Could you check a few things on this model? Use its own coordinates, in mm. A direction names the side the tool comes from. Round coordinates to 2 decimals unless told otherwise and drop trailing zeros. Loops run counter-clockwise (first coordinate to the right, second up) from the corner with the lowest first, then second, coordinate; pieces in that order, holes last. Notation, with made-up numbers: (74.5, -3.75) -> (82.5, -3.75) arc R22 ccw to (82.5, 31.25) -> close; hole circle Ø7 at (-22, 61.25). An arc over 180 degrees is marked (long way). Write each question's results on one line, items separated by ' | '.
from build123d import *

# Parameters (mm, degrees)
F1_DEPTH = 10
F2_W     = 8
F2_H     = 1.25
F3_DEPTH = 25
F4_W     = 0.5
F4_H     = 0.5
F5_DEPTH = 25
F6_W     = 6
F6_H     = 1
F7_DEPTH = 1


with BuildPart() as f1:
    # F0 (on Top) → F1 (new body)
    with BuildSketch(Plane.XY):
        Polygon((0, 3.5), (0, 0), (6, 0), (6, 11.5), (5, 11.5), (5, 3.5), align=None)
    extrude(amount=F1_DEPTH)

    # F2 (on face) → F3 (cut)
    with BuildSketch(Plane(origin=(5, 0, 0), x_dir=(0, -1, 0), z_dir=(-1, 0, 0))):
        with Locations((-7.5, 0.625)):
            Rectangle(F2_W, F2_H)
        with Locations((-7.5, 9.375)):
            Rectangle(F2_W, F2_H)
    extrude(amount=-F3_DEPTH, mode=Mode.SUBTRACT)

    # F4 (on face) → F5 (cut)
    with BuildSketch(Plane.XZ):
        with Locations((3.75, 8.5)):
            Rectangle(F4_W, F4_H)
        with Locations((3.75, 1.5)):
            Rectangle(F4_W, F4_H)
        with Locations((3.75, 6.166667)):
            Rectangle(F4_W, F4_H)
        with Locations((3.75, 3.833333)):
            Rectangle(F4_W, F4_H)
    extrude(amount=-F5_DEPTH, mode=Mode.SUBTRACT)

    # F6 (on face) → F7 (cut)
    with BuildSketch(Plane.XZ):
        with Locations((3, 8.5)):
            Rectangle(F6_W, F6_H)
        with Locations((3, 6.166667)):
            Rectangle(F6_W, F6_H)
        with Locations((3, 3.833333)):
            Rectangle(F6_W, F6_H)
        with Locations((3, 1.5)):
            Rectangle(F6_W, F6_H)
    extrude(amount=-F7_DEPTH, mode=Mode.SUBTRACT)


solid = f1.part
1) I want a section at D-D, the plane y = 3.75. Write out the boundary of the cut face in (x, z).
Model answer:
outline: (5, 1.25) -> (6, 1.25) -> (6, 8.75) -> (5, 8.75) -> close
2) I want a section at B-B, the plane z = 7. Write out the boundary of the cut face in (x, y).
Model answer:
outline: (0, 0) -> (6, 0) -> (6, 11.5) -> (5, 11.5) -> (5, 3.5) -> (0, 3.5) -> close
3) I'm going to push flat-ended pins straight in: pin 1 (0.8 mm diameter, centred on x = 5.5, y = 9, fed in from -Z); pin 2 (3 mm diameter, centred on y = 6.5, z = 9, fed in from -X); pin 3 (0.8 mm diameter, centred on x = 4.5, z = 1.5, fed in from -Y). Where does each tip first touch, or does it pass through?
Model answer:
pin 1: stops at z = 1.25 | pin 2: stops at x = 5 | pin 3: stops at y = 1
4) For faces 4 (the flat face through (3, 0.5, 5.667)), 5 (the flat face through (3, 0, 3)), 6 (the flat face through (5.5, 7.6, 8.75)), which set-ups out of +Z, -Z, +X, -X, +Y, -Y let a thin tool reach every point of the face, with its end or its side?
Model answer:
face 4: +X, -X, -Y | face 5: +Z, -Z, +X, -X, -Y | face 6: +Z, +X, -X, +Y
5) If we mould it in two halves opening along Z, with no side actions, what happens to faces 1 (the flat face through (3, 0.5, 8)), 2 (the flat face through (5, 8, 5)), 3 (the flat face through (5.5, 7.6, 1.25))? For each: released by +Z, released by -Z, zero draft, split by the parting line, or undercut.
Model answer:
face 1: undercut | face 2: zero draft | face 3: released by -Z
6) I need wall thicknesses on line 1 (Z direction, x = 5.3, y = 0.5); line 2 (Y direction, x = 1.65, z = 2.5); line 3 (Z direction, x = 5.35, y = 3.75). Which ranges of each line are inside material? Lowest first, please.
Model answer:
line 1: z = 0 to 1, 2 to 3.33, 4.33 to 5.67, 6.67 to 8, 9 to 10 | line 2: y = 0 to 3.5 | line 3: z = 1.25 to 8.75
7) I want a section at A-A, the plane x = 1.6. Write out the boundary of the cut face in (y, z), plus the area to 3 significant figures.
Model answer:
outline: (0, 0) -> (3.5, 0) -> (3.5, 10) -> (0, 10) -> (0, 9) -> (1, 9) -> (1, 8) -> (0, 8) -> (0, 6.67) -> (1, 6.67) -> (1, 5.67) -> (0, 5.67) -> (0, 4.33) -> (1, 4.33) -> (1, 3.33) -> (0, 3.33) -> (0, 2) -> (1, 2) -> (1, 1) -> (0, 1) -> close | area: 31.0 mm2
8) I want a section at C-C, the plane x = 3.7. Give the number of separate pieces and of enclosed holes in the cut face, plus the area to 3 significant figures.
Model answer:
separate pieces: 5 | enclosed holes: 0 | area: 26.0 mm2
